```python
from build123d import *

# Parameters (mm, degrees)
SKETCH_1_W           = 55
SKETCH_1_H           = 29
EXTRUDE_1_DEPTH      = 13
SKETCH_2_OUTSIDE_W   = 69.704
SKETCH_2_OUTSIDE_H   = 43.704
SKETCH_2_OUTSIDE_W_2 = 55
SKETCH_2_OUTSIDE_H_2 = 29
SKETCH_2_OUTSIDE_R   = 4
CUT_EXTRUDE_1_DEPTH  = 13
FILLET_1_R           = 10


with BuildPart() as part:
    # 草图1 → 凸台-拉伸1 (new body)
    with BuildSketch(Plane.XY):
        with Locations((3.176056338, -2.774647887)):
            Rectangle(SKETCH_1_W, SKETCH_1_H)
    extrude(amount=EXTRUDE_1_DEPTH)

    # 草图2 outside → 切除-拉伸1 (cut)
    with BuildSketch(Plane.XY.offset(13)):
        with Locations((3.176, -2.775)):
            Rectangle(SKETCH_2_OUTSIDE_W, SKETCH_2_OUTSIDE_H)
        with Locations((3.176056338, -2.774647887)):
            Rectangle(SKETCH_2_OUTSIDE_W_2, SKETCH_2_OUTSIDE_H_2, mode=Mode.SUBTRACT)
        with Locations((3.176056338, -2.274647887)):
            Circle(SKETCH_2_OUTSIDE_R)
    extrude(amount=-CUT_EXTRUDE_1_DEPTH, mode=Mode.SUBTRACT)

    # 圆角1
    fillet_1_edges = [part.edges().sort_by_distance(p)[0] for p in [
        (-24.323943662, 11.725352113, 6.5),
        (30.676056338, 11.725352113, 6.5),
    ]]
    fillet(fillet_1_edges, radius=FILLET_1_R)


solid = part.part
```
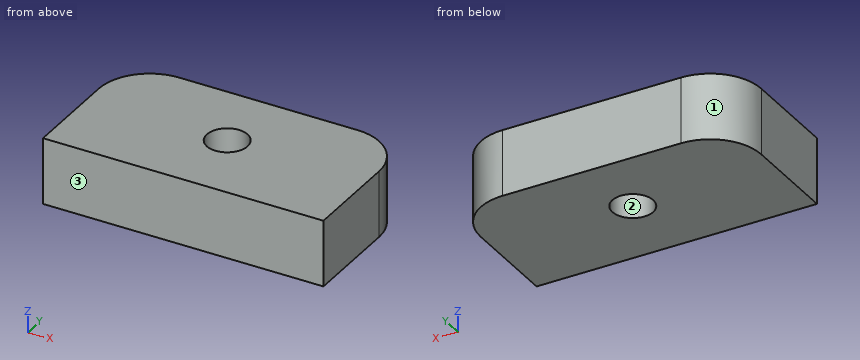
Read the model definition and answer for the solid it produces. Units are mm, in the model's axes. Face numbers are marked on the shaded views. Give positions to 0.01 mm unless a question says otherwise; leave off trailing zeros. Write each loop counter-clockwise with the first axis right and the second up, starting at its lowest first coordinate (ties: lowest second). Pieces come first, ordered by that corner, then holes. Notation, with made-up numbers: (35.5, 81.25) - (63.5, 81.25) arc R12 cw to (63.5, 95.25) - close; hole circle Ø9 at (-17, -35.75). An arc over 180 degrees is marked (long way). Write item = value, one per line. Start each with the question number.
Item 1: Find section B-B (z = 1.25). Give the vertices of the cut face in (x, y), then the cut area to 3 significant figures.
Item 2: The mould has two halves that part along X. Classify the marked faces 1, 2 and 3: +X half, -X half, draft (parallel to the pull), parting line (faces both ways), or undercut.
Item 3: Find section C-C (x = 6). Give the vertices of the cut face in (y, z).
Item 4: Find the intervals of material crossed by probe 1 along X at (y, z) = (-2.5, 2.75); probe 2 along Y at (x, z) = (2, 3.75); probe 3 along Y at (x, z) = (1, 10.25), in increasing order. Write a range as [from, to].
Item 5: Find section D-D (y = 10). Give the vertices of the cut face in (x, z), then the cut area to 3 significant figures.
Item 6: Find section A-A (y = 0). Give the vertices of the cut face in (x, z).
Response:
q1.outline = (-24.32, -17.27) - (30.68, -17.27) - (30.68, 1.73) arc R10 ccw to (20.68, 11.73) - (-14.32, 11.73) arc R10 ccw to (-24.32, 1.73) - close; hole circle Ø8 at (3.18, -2.27)
q1.area = 1,500 mm²
q2.face_1 = -X half
q2.face_2 = undercut
q2.face_3 = draft
q3.outline = (-17.27, 0) - (-5.11, 0) - (-5.11, 13) - (-17.27, 13) - close; (0.56, 0) - (11.73, 0) - (11.73, 13) - (0.56, 13) - close
q4.probe_1 = [-24.32, -0.82], [7.17, 30.68]
q4.probe_2 = [-17.27, -6.1], [1.55, 11.73]
q4.probe_3 = [-17.27, -5.63], [1.08, 11.73]
q5.outline = (-19.94, 0) - (26.29, 0) - (26.29, 13) - (-19.94, 13) - close
q5.area = 601 mm²
q6.outline = (-24.32, 0) - (-0.11, 0) - (-0.11, 13) - (-24.32, 13) - close; (6.47, 0) - (30.68, 0) - (30.68, 13) - (6.47, 13) - close
